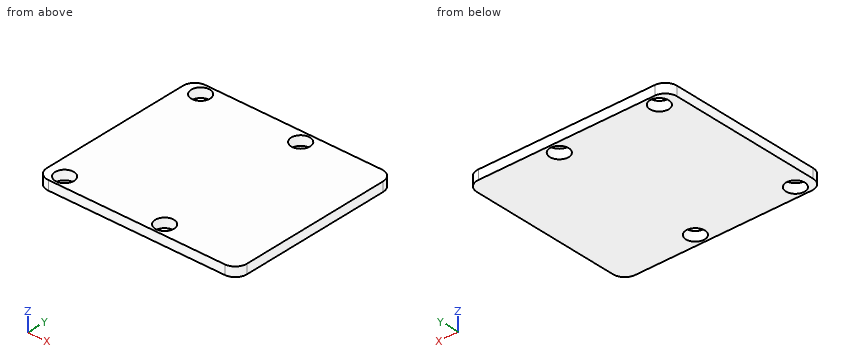
```python
from build123d import *

# Parameters (mm, degrees)
SKETCH1_W           = 34
SKETCH1_H           = 30
BOSS_EXTRUDE1_DEPTH = 1.6
CUT_EXTRUDE1_REACH  = 24.728
SKETCH2_R           = 1.6
FILLET1_R           = 2


with BuildPart() as part:
    # Sketch1 → Boss-Extrude1 (new body)
    with BuildSketch(Plane.XY):
        Rectangle(SKETCH1_W, SKETCH1_H)
    extrude(amount=BOSS_EXTRUDE1_DEPTH)

    # Sketch2 → Cut-Extrude1 (cut, up to next)
    with BuildSketch(Plane.XY, mode=Mode.PRIVATE) as cut_extrude1_sk1:
        with Locations((-14, 13)):
            Circle(SKETCH2_R)
    cut_extrude1_tool1 = extrude(cut_extrude1_sk1.sketch, amount=CUT_EXTRUDE1_REACH, mode=Mode.PRIVATE) & part.part
    # Sketch2 → Cut-Extrude1 (cut, up to next)
    with BuildSketch(Plane.XY, mode=Mode.PRIVATE) as cut_extrude1_sk2:
        with Locations((3, 13)):
            Circle(SKETCH2_R)
    cut_extrude1_tool2 = extrude(cut_extrude1_sk2.sketch, amount=CUT_EXTRUDE1_REACH, mode=Mode.PRIVATE) & part.part
    # Sketch2 → Cut-Extrude1 (cut, up to next)
    with BuildSketch(Plane.XY, mode=Mode.PRIVATE) as cut_extrude1_sk3:
        with Locations((3, -13)):
            Circle(SKETCH2_R)
    cut_extrude1_tool3 = extrude(cut_extrude1_sk3.sketch, amount=CUT_EXTRUDE1_REACH, mode=Mode.PRIVATE) & part.part
    # Sketch2 → Cut-Extrude1 (cut, up to next)
    with BuildSketch(Plane.XY, mode=Mode.PRIVATE) as cut_extrude1_sk4:
        with Locations((-14, -13)):
            Circle(SKETCH2_R)
    cut_extrude1_tool4 = extrude(cut_extrude1_sk4.sketch, amount=CUT_EXTRUDE1_REACH, mode=Mode.PRIVATE) & part.part
    add(cut_extrude1_tool1.solids().sort_by_distance((-14, 13, 0))[0], mode=Mode.SUBTRACT)
    add(cut_extrude1_tool2.solids().sort_by_distance((3, 13, 0))[0], mode=Mode.SUBTRACT)
    add(cut_extrude1_tool3.solids().sort_by_distance((3, -13, 0))[0], mode=Mode.SUBTRACT)
    add(cut_extrude1_tool4.solids().sort_by_distance((-14, -13, 0))[0], mode=Mode.SUBTRACT)

    # Fillet1
    fillet1_edges = [part.edges().sort_by_distance(p)[0] for p in [
        (17, -15, 0.8),
        (-17, -15, 0.8),
        (-17, 15, 0.8),
        (17, 15, 0.8),
    ]]
    fillet(fillet1_edges, radius=FILLET1_R)


solid = part.part
```
Check sheet for the modelled part. Datum: model origin and axes. Units: mm. Give positions to 0.01 mm unless a question says otherwise; leave off trailing zeros. Order: outer loops, then holes, each group sorted by start corner. A loop starts at its lowest first (then second) coordinate and runs counter-clockwise, first axis right, second up. Notation, with made-up numbers: M 79.25,-39.5 L 118.25,-39.5 A8 ccw 118.25,-27.5 Z; hole C -23,-20 d3. An arc over 180 degrees is marked long. Answer in a Markdown table with one row per item. Add a question column.
Q1. Thickness scan on L1, parallel to X at y = -13, z = 0.65; L2, parallel to Y at x = 3, z = 0.8; L3, parallel to X at y = -11.75, z = 0.5. Record the ranges inside material, lowest first.
Q2. Sectioned sample at C-C, the plane y = -12.25. Record the boundary of the cut face in (x, z), and give its area (3 significant figures).
Q3. Sectioned sample at A-A, the plane x = -14. Record the boundary of the cut face in (y, z), and give its area (3 significant figures).
Q4. Gauge pin test, flat end, axial feed: pin 1 Ø4 at (x, y) = (3, -13) entering from -Z. Record the tip position at first contact, or that the pin passes through.
Q5. Sectioned sample at B-B, the plane z = 0.5. Record the boundary of the cut face in (x, y), and give its area (3 significant figures).
Verdict:
| question | item | result |
|---|---|---|
| 1 | L1 | -17 to -15.6, -12.4 to 1.4, 4.6 to 17 |
| 1 | L2 | -15 to -14.6, -11.4 to 11.4, 14.6 to 15 |
| 1 | L3 | -17 to -15, -13 to 2, 4 to 17 |
| 2 | outline | M -17,0 L -15.41,0 L -15.41,1.6 L -17,1.6 Z; M -12.59,0 L 1.59,0 L 1.59,1.6 L -12.59,1.6 Z; M 4.41,0 L 17,0 L 17,1.6 L 4.41,1.6 Z |
| 2 | area | 45.4 mm² |
| 3 | outline | M -15,0 L -14.6,0 L -14.6,1.6 L -15,1.6 Z; M -11.4,0 L 11.4,0 L 11.4,1.6 L -11.4,1.6 Z; M 14.6,0 L 15,0 L 15,1.6 L 14.6,1.6 Z |
| 3 | area | 37.8 mm² |
| 4 | pin 1 | z = 0 |
| 5 | outline | M -17,-13 A2 ccw -15,-15 L 15,-15 A2 ccw 17,-13 L 17,13 A2 ccw 15,15 L -15,15 A2 ccw -17,13 Z; hole C -14,-13 d3.2; hole C -14,13 d3.2; hole C 3,-13 d3.2; hole C 3,13 d3.2 |
| 5 | area | 984 mm² |
